Read the model definition and answer for the solid it produces. Units are mm, in the model's axes. A direction names the side the tool comes from. Round coordinates to 2 decimals unless told otherwise and drop trailing zeros. Order: outer loops, then holes, each group sorted by start corner. A loop starts at its lowest first (then second) coordinate and runs counter-clockwise, first axis right, second up. Notation, with made-up numbers: (-29.5, 50.5) -> (-7.5, 50.5) arc R13 cw to (-7.5, 75.5) -> close; hole circle Ø6 at (-5, 82). An arc over 180 degrees is marked (long way). Answer as a JSON object with one key per item and string values. Group by question number.
Item 1: The mould has two halves that part along Y. Classify faces 3 (the flat face through (723.9, -3, 0)), 4 (the flat face through (-10, 203.2, 0)): pulls with the +Y half, pulls with the -Y half, needs draft (parallel to the pull), parting line crosses it, or undercut.
Item 2: Given P1, Ø2, axis at x = -561.5, z = 9.5, coming from the -Y side; P2, Ø10, axis at x = -565, z = 7, coming from the +Y side; P3, Ø7.5, axis at y = -210.82, z = 0.15, coming from the +X side; P4, Ø1, axis at x = -162.5, z = 3.5, coming from the -Y side, each flat-ended and moving along its own axis, determine where each tip first touches the part or whether it passes through.
Item 3: Section B-B, the plane x = -172 is taken. Write down the section's boundary in (y, z), plus the area to 3 significant figures.
Item 4: For faces 1 (the flat face through (-10, -203.2, 0)), 2 (the flat face through (-10, 3, 12.7)), determine the directions among +Z, -Z, +X, -X, +Y, -Y from which every point of the face is accessible in a straight line to the end or side of a thin tool.
Item 5: Section A-A, the plane x = 519 is taken. Write down the section's boundary in (y, z) (3 decimals).
Item 6: Consider probe 1 along Y at (x, z) = (-418.5, 1); probe 2 along Z at (x, y) = (-464.5, 210.82) (3 decimals); probe 3 along Y at (x, z) = (580, -3.75). Determine where each line is inside the solid, lowest interval first. Write a range as from..to.
from build123d import *

# Parameters (mm, degrees)
F0_W     = 1447.8
F0_H     = 406.4
F5_DEPTH = 12.7
F4_R     = 9.525
F4_R_2   = 6.35
F6_DEPTH = 361.95
F3_R     = 9.525
F3_R_2   = 6.35
F7_DEPTH = 361.95
F8_DEPTH = 361.95
F9_DEPTH = 361.95


with BuildPart() as f5:
    # F0 (on Top) → F5 (new body, symmetric)
    with BuildSketch(Plane.XY):
        Rectangle(F0_W, F0_H)
    extrude(amount=F5_DEPTH, both=True)

    # F4 (on offset) → F6 (join)
    with BuildSketch(Plane.YZ.offset(-361.95)):
        with Locations((210.82, 0)):
            Circle(F4_R)
        with Locations((210.82, 0)):
            Circle(F4_R_2, mode=Mode.SUBTRACT)
    extrude(amount=-F6_DEPTH)

    # F3 (on offset) → F7 (join)
    with BuildSketch(Plane.YZ.offset(361.95)):
        with Locations((210.82, 0)):
            Circle(F3_R)
        with Locations((210.82, 0)):
            Circle(F3_R_2, mode=Mode.SUBTRACT)
    extrude(amount=F7_DEPTH)

    # F4 (on offset) → F8 (join)
    with BuildSketch(Plane.YZ.offset(-361.95)):
        with Locations((-210.82, 0.1492979936)):
            Circle(F4_R)
        with Locations((-210.82, 0.1492979936)):
            Circle(F4_R_2, mode=Mode.SUBTRACT)
    extrude(amount=-F8_DEPTH)

    # F3 (on offset) → F9 (join)
    with BuildSketch(Plane.YZ.offset(361.95)):
        with Locations((-210.82, -0.1084019023)):
            Circle(F3_R)
        with Locations((-210.82, -0.1084019023)):
            Circle(F3_R_2, mode=Mode.SUBTRACT)
    extrude(amount=F9_DEPTH)


solid = f5.part
Values found:
{
 "1": {"face 3": "needs draft", "face 4": "undercut"},
 "2": {"P1": "y = -215.4", "P2": "y = 220.13", "P3": "through", "P4": "y = -203.2"},
 "3": {"outline": "(-203.2, -12.7) -> (203.2, -12.7) -> (203.2, 12.7) -> (-203.2, 12.7) -> close", "area": "10,300 mm2"},
 "4": {"face 1": "none", "face 2": "+Z, +X, -X, +Y, -Y"},
 "5": {"outline": "(-203.2, -12.7) -> (203.2, -12.7) -> (203.2, -5.715) arc R9.525 ccw (long way) to (203.2, 5.715) -> (203.2, 12.7) -> (-203.2, 12.7) -> (-203.2, 5.607) arc R9.525 ccw (long way) to (-203.2, -5.823) -> close; hole circle Ø12.7 at (-210.82, -0.108); hole circle Ø12.7 at (210.82, 0)"},
 "6": {"probe 1": "-220.31..-217.11, -204.53..204.55, 217.09..220.29", "probe 2": "-9.525..-6.35, 6.35..9.525", "probe 3": "-219.62..-216.02, -205.62..205.7, 215.94..219.58"}
}
